Verification items for the finished model (mm, model axes). Coordinates: 2 decimals unless noted, no trailing zeros. Order: outer loops, then holes, each group sorted by start corner. A loop starts at its lowest first (then second) coordinate and runs counter-clockwise, first axis right, second up. Notation, with made-up numbers: (22.5, 17) -> (38.5, 17) arc R21 cw to (38.5, 50) -> close; hole circle Ø5 at (52.5, -20). An arc over 180 degrees is marked (long way). Write each question's results on one line, items separated by ' | '. Start each with the question number.
(1) Cross-section at A-A on y = -126.5. Enter the section's corners in (x, z).
(2) Cross-section at B-B on z = -22.5. Enter the section's corners in (x, y).
(3) Thickness scan on probe 1 along X at (y, z) = (-131.5, -22.85); probe 2 along Y at (x, z) = (0, -22.7); probe 3 along X at (y, z) = (-124.25, -22.3). Record the ranges inside material, lowest first. Write a range as [from, to].
```python
from build123d import *

# Parameters (mm, degrees)
SKETCH028_W  = 10
SKETCH028_H  = 25
PAD015_DEPTH = 1
FILLET021_R  = 2
FILLET022_R  = 0.9


with BuildPart() as part:
    # Sketch028 → Pad015 (new body)
    with BuildSketch(Plane.XY):
        Rectangle(SKETCH028_W, SKETCH028_H)
    extrude(amount=PAD015_DEPTH)

    # Fillet021
    fillet021_edges = [part.edges().sort_by_distance(p)[0] for p in [
        (-5, -12.5, 0.5),
        (-5, 12.5, 0.5),
        (5, -12.5, 0.5),
        (5, 12.5, 0.5),
    ]]
    fillet(fillet021_edges, radius=FILLET021_R)

    # Fillet022
    fillet022_edges = [part.edges().sort_by_distance(p)[0] for p in [
        (0, -12.5, 1),
        (5, 0, 1),
        (-5, 0, 1),
        (0, 12.5, 1),
    ]]
    fillet(fillet022_edges, radius=FILLET022_R)


with BuildPart() as part_1:
    # Body007 placement: moved
    add(part.part.moved(Location((0, -130, -23))))


solid = part_1.part
```
Results are:
1) outline: (-5, -23) -> (5, -23) -> (5, -22.9) arc R0.9 ccw to (4.1, -22) -> (-4.1, -22) arc R0.9 ccw to (-5, -22.9) -> close
2) outline: (-4.91, -140.5) arc R1.91 ccw to (-3, -142.41) -> (3, -142.41) arc R1.91 ccw to (4.91, -140.5) -> (4.91, -119.5) arc R1.91 ccw to (3, -117.59) -> (-3, -117.59) arc R1.91 ccw to (-4.91, -119.5) -> close
3) probe 1: x = [-5, 5] | probe 2: y = [-142.48, -117.52] | probe 3: x = [-4.77, 4.77]
